```python
from build123d import *

# Parameters (mm, degrees)
F0_W     = 304.8
F0_H     = 457.2
F1_DEPTH = 50.8
F2_W     = 76.2
F2_H     = 75.8903771639
F2_H_2   = 75.2589152813
F3_DEPTH = 50.8
F4_DEPTH = 50.8
F5_DEPTH = 50.8
F6_DEPTH = 50.8


with BuildPart() as f1:
    # F0 (on Top) → F1 (new body)
    with BuildSketch(Plane.XY):
        Rectangle(F0_W, F0_H)
    extrude(amount=F1_DEPTH)

    # F2 (on face) → F3 (join)
    with BuildSketch(Plane.XY.offset(50.8)):
        Polygon((-38.1, 0), (0, 0), (38.1, 0), (38.1, 77.4507075548), (-38.1, 77.4507075548), align=None)
        with BuildLine():
            Line((38.1, 0), (0, 0))
            Line((0, 0), (-38.1, 0))
            Line((-38.1, 0), (-38.1, -212.1318222238))
            ThreePointArc((-38.1, -212.1318222238), (-19.4052442067, -221.1877873667), (0, -228.6))
            ThreePointArc((0, -228.6), (19.4052442067, -221.1877873667), (38.1, -212.1318222238))
            Line((38.1, -212.1318222238), (38.1, 0))
        make_face()
        with Locations((0, 115.3958961368)):
            Rectangle(F2_W, F2_H)
        with BuildLine():
            Line((38.1, -228.6), (38.1, -212.1318222238))
            ThreePointArc((38.1, -212.1318222238), (19.4052442067, -221.1877873667), (0, -228.6))
            Line((0, -228.6), (38.1, -228.6))
        make_face()
        with BuildLine():
            ThreePointArc((0, -228.6), (-19.4052442067, -221.1877873667), (-38.1, -212.1318222238))
            Line((-38.1, -212.1318222238), (-38.1, -228.6))
            Line((-38.1, -228.6), (0, -228.6))
        make_face()
        with Locations((0, 190.9705423594)):
            Rectangle(F2_W, F2_H_2)
        with BuildLine():
            Line((76.2, 0), (38.1, 0))
            Line((38.1, 0), (38.1, -212.1318222238))
            ThreePointArc((38.1, -212.1318222238), (108.2301156896, -155.0804063276), (152.4, -76.2))
            Line((152.4, -76.2), (152.4, 0))
            Line((152.4, 0), (76.2, 0))
        make_face()
    extrude(amount=-F3_DEPTH)

    # F2 (on face) → F4 (cut)
    with BuildSketch(Plane.XY.offset(50.8)):
        with BuildLine():
            ThreePointArc((0, -228.6), (-19.4052442067, -221.1877873667), (-38.1, -212.1318222238))
            Line((-38.1, -212.1318222238), (-38.1, -228.6))
            Line((-38.1, -228.6), (0, -228.6))
        make_face()
        with BuildLine():
            Line((-38.1, -228.6), (-38.1, -212.1318222238))
            ThreePointArc((-38.1, -212.1318222238), (-108.2301156896, -155.0804063276), (-152.4, -76.2))
            Line((-152.4, -76.2), (-152.4, -228.6))
            Line((-152.4, -228.6), (-38.1, -228.6))
        make_face()
    extrude(amount=-F4_DEPTH, mode=Mode.SUBTRACT)

    # F2 (on face) → F5 (cut)
    with BuildSketch(Plane.XY.offset(50.8)):
        with BuildLine():
            Line((38.1, -228.6), (38.1, -212.1318222238))
            ThreePointArc((38.1, -212.1318222238), (19.4052442067, -221.1877873667), (0, -228.6))
            Line((0, -228.6), (38.1, -228.6))
        make_face()
        with BuildLine():
            ThreePointArc((152.4, -76.2), (108.2301156896, -155.0804063276), (38.1, -212.1318222238))
            Line((38.1, -212.1318222238), (38.1, -228.6))
            Line((38.1, -228.6), (152.4, -228.6))
            Line((152.4, -228.6), (152.4, -76.2))
        make_face()
    extrude(amount=-F5_DEPTH, mode=Mode.SUBTRACT)

    # F2 (on face) → F6 (cut)
    with BuildSketch(Plane.XY.offset(50.8)):
        with BuildLine():
            Line((-38.1, -228.6), (-38.1, -212.1318222238))
            ThreePointArc((-38.1, -212.1318222238), (-108.2301156896, -155.0804063276), (-152.4, -76.2))
            Line((-152.4, -76.2), (-152.4, -228.6))
            Line((-152.4, -228.6), (-38.1, -228.6))
        make_face()
        with BuildLine():
            ThreePointArc((152.4, -76.2), (108.2301156896, -155.0804063276), (38.1, -212.1318222238))
            Line((38.1, -212.1318222238), (38.1, -228.6))
            Line((38.1, -228.6), (152.4, -228.6))
            Line((152.4, -228.6), (152.4, -76.2))
        make_face()
    extrude(amount=-F6_DEPTH, mode=Mode.SUBTRACT)


solid = f1.part
```
Read the model definition and answer for the solid it produces. Units are mm, in the model's axes. Round coordinates to 2 decimals unless told otherwise and drop trailing zeros. Write each loop counter-clockwise with the first axis right and the second up, starting at its lowest first coordinate (ties: lowest second). Pieces come first, ordered by that corner, then holes. Notation, with made-up numbers: (30.25, 56.5) - (78.25, 56.5) arc R9 cw to (78.25, 73.5) - close; hole circle Ø7 at (51.25, -36). An arc over 180 degrees is marked (long way). One line per item, written item: value.
Q1. Find section C-C (x = 68). Determine the outline of the cut face in (y, z).
The answers:
outline: (-193.06, 0) - (228.6, 0) - (228.6, 50.8) - (-193.06, 50.8) - close
Q2. Find section A-A (z = 17). Determine the outline of the cut face in (x, y).
The answers:
outline: (-152.4, -76.2) arc R240.97 ccw to (0, -228.6) arc R240.97 ccw to (152.4, -76.2) - (152.4, 228.6) - (-152.4, 228.6) - close
Q3. Find section B-B (y = -146). Determine the outline of the cut face in (x, z).
The answers:
outline: (-115.5, 0) - (115.5, 0) - (115.5, 50.8) - (-115.5, 50.8) - close
Q4. Straight lines are drawn through the part: line 1 (Y direction, x = -3, z = 20.5); line 2 (Y direction, x = -14, z = 20); line 3 (X direction, y = -178, z = 22). For each, find the intervals that lie inside material, in ascending order. Write a range as from..to.
The answers:
line 1: y = -227.58..228.6
line 2: y = -223.45..228.6
line 3: x = -86.22..86.22
Q5. Each of these flat-tipped pins is pushed along its axis until it touches: P1, Ø5, axis at x = -14.5, z = 9.5, coming from the -Y side; P2, Ø6, axis at x = -109, z = 31.5, coming from the -Y side; P3, Ø8, axis at x = -18, y = 27, coming from the -Z side. Where does it stop, or does it pass through?
The answers:
P1: stops at y = -224.24
P2: stops at y = -157.69
P3: stops at z = 0
